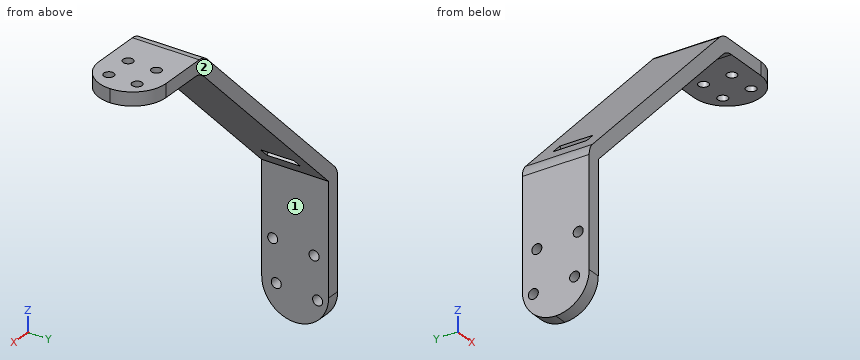
```python
from build123d import *

# Parameters (mm, degrees)
F1_DEPTH = 20
F3_R     = 9.99999
F4_D     = 3
F5_R     = 5
F7_D     = 3
F8_W     = 4
F8_H     = 10
F9_DEPTH = 25


# Not quite as in the source:
# - a fillet or chamfer is up to 0.001 mm smaller than in the source, because OpenCascade refuses the exact size


with BuildPart() as f1:
    # F0 (on Front) → F1 (new body)
    with BuildSketch(Plane.XZ):
        Polygon((-4, 0), (0, 0), (0, 43), (56.5685424949, 99.5685424949), (81.5685424949, 99.5685424949), (81.5685424949, 103.5685424949), (54.9116882454, 103.5685424949), (-4, 44.6568542495), align=None)
    extrude(amount=F1_DEPTH)

    # F3 (radius 10 in the source; OpenCascade refuses exactly that, so slightly less here)
    f3_edges = [f1.edges().sort_by_distance(p)[0] for p in [
        (-2, -20, 0),
        (-2, 0, 0),
        (81.568542, 0, 101.568542),
        (81.568542, -20, 101.568542),
    ]]
    fillet(f3_edges, radius=F3_R)

    # F4 (through all)
    with Locations(Plane(origin=(0, 0, 99.5685424949), x_dir=(1, 0, 0), z_dir=(0, 0, -1))):
        with Locations((75.811183182, 14.2426406871), (67.3259018078, 14.2426406871), (67.3259018078, 5.7573593129), (75.811183182, 5.7573593129)):
            Hole(F4_D / 2)

    # F5
    f5_edges = [f1.edges().sort_by_distance(p)[0] for p in [
        (54.911688, -10, 103.568542),
        (56.568542, -10, 99.568542),
        (-4, -10, 44.656854),
    ]]
    fillet(f5_edges, radius=F5_R)

    # F7 (through all)
    with Locations(Plane.YZ):
        with Locations((-4.3431457505, 20.6568542495), (-16.7175144213, 21.7175144213), (-15.6568542495, 9.3431457505), (-3.2824855787, 8.2824855787)):
            Hole(F7_D / 2)

    # F8 (on face) → F9 (cut)
    with BuildSketch(Plane(origin=(-21.5, 0, 21.5), x_dir=(0.7071067812, 0, 0.7071067812), z_dir=(0.7071067812, 0, -0.7071067812))):
        with Locations((39.5918783247, 10)):
            Rectangle(F8_W, F8_H)
    extrude(amount=-F9_DEPTH, mode=Mode.SUBTRACT)


solid = f1.part
```
Work out the finished part from the listing and answer in its coordinate system (mm). Face numbers are marked on the shaded views. A direction names the side the tool comes from. Give positions to 0.01 mm unless a question says otherwise; leave off trailing zeros. Write each loop counter-clockwise with the first axis right and the second up, starting at its lowest first coordinate (ties: lowest second). Pieces come first, ordered by that corner, then holes.
(1) Straight lines are drawn through the part: line 1 (Z direction, x = 69.5, y = -7); line 2 (X direction, y = -15.25, z = 5); line 3 (X direction, y = -3.75, z = 86.5). For each, find the intervals that lie inside material, in ascending order.
Final values:
line 1: z = 99.57 to 103.57
line 2: x = -4 to 0
line 3: x = 37.84 to 43.5
(2) Which of the six approach directions +Z, -Z, +X, -X, +Y, -Y give full straight-line access (tool end or side, diameter ignored) to the marked faces 1 and 2?
Final values:
face 1: -Z, +X, +Y, -Y
face 2: +Z, -Z, +X, -X, +Y
(3) The part is cut by section B-B on y = -8.75. Write down the section's boundary in (x, z).
Final values:
outline: (-4, 0.08) - (0, 0.08) - (0, 43) - (5.08, 48.08) - (2.25, 50.91) - (-2.54, 46.12) arc R5 ccw to (-4, 42.59) - close; (5.08, 53.74) - (7.91, 50.91) - (55.1, 98.1) arc R5 cw to (58.64, 99.57) - (81.49, 99.57) - (81.49, 103.57) - (56.98, 103.57) arc R5 ccw to (53.45, 102.1) - close
(4) The part is cut by section A-A on x = 76. Write down the section's boundary in (y, z).
Final values:
outline: (-18.96, 99.57) - (-15.73, 99.57) - (-15.73, 103.57) - (-18.96, 103.57) - close; (-12.75, 99.57) - (-7.25, 99.57) - (-7.25, 103.57) - (-12.75, 103.57) - close; (-4.27, 99.57) - (-1.04, 99.57) - (-1.04, 103.57) - (-4.27, 103.57) - close
(5) The part is cut by section D-D on z = 37.5. Write down the section's boundary in (x, y), plus the area to 3 significant figures.
Final values:
outline: (-4, -20) - (0, -20) - (0, 0) - (-4, 0) - close
area: 80.0 mm2
(6) Flat-ended cylindrical pins translate along their axes: pin 1 Ø5 at (y, z) = (-17, 45) entering from +X; pin 2 Ø5 at (x, y) = (75.81, -14.24) entering from +Z; pin 3 Ø1 at (x, y) = (25.5, -16.5) entering from -Z; pin 4 Ø4 at (y, z) = (-15.66, 9.34) entering from +X. Find the tip coordinate at first contact, or state that the pin passes through.
Final values:
pin 1: stops at x = 4.5
pin 2: stops at z = 103.57
pin 3: stops at z = 68
pin 4: stops at x = 0
(7) The part is cut by section C-C on x = 60.5. Write down the section's boundary in (y, z), plus the area to 3 significant figures.
Final values:
outline: (-20, 99.57) - (0, 99.57) - (0, 103.57) - (-20, 103.57) - close
area: 80.0 mm2
